Work out the finished part from the listing and answer in its coordinate system (mm). Face numbers are marked on the shaded views. A direction names the side the tool comes from. Coordinates: 2 decimals unless noted, no trailing zeros. Order: outer loops, then holes, each group sorted by start corner. A loop starts at its lowest first (then second) coordinate and runs counter-clockwise, first axis right, second up. Notation, with made-up numbers: M 22.5,-20 L 80.5,-20 A17 cw 80.5,-8 Z; hole C 43,60 d4. An arc over 180 degrees is marked long. Use a Markdown table: item, result.
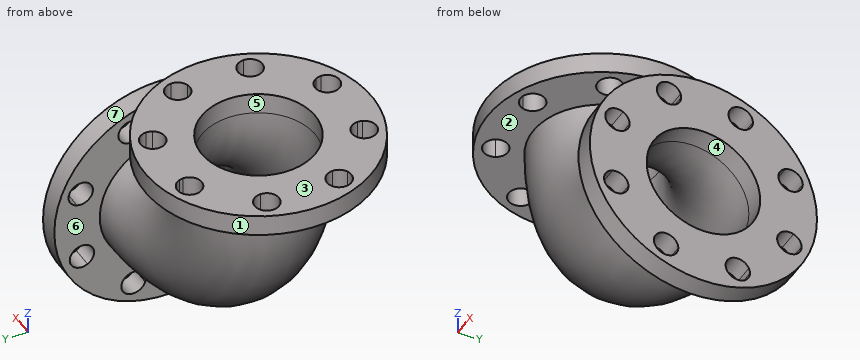
from build123d import *

# Parameters (mm, degrees)
F0_R     = 127
F0_R_2   = 76.2
F0_R_3   = 63.5
F1_DEPTH = 23.8125
F2_ANGLE = 90
F3_R     = 127
F3_R_2   = 76.2
F3_R_3   = 63.5
F4_DEPTH = 23.8125


with BuildPart() as f1:
    # F0 (on Top) → F1 (new body)
    with BuildSketch(Plane.XY):
        Circle(F0_R)
        with BuildLine():
            ThreePointArc((28.8603537964, 100.7217980566), (44.0561876825, 109.567966691), (55.3745369645, 96.1120001135))
            ThreePointArc((55.3745369645, 96.1120001135), (54.9915876268, 92.9004802457), (53.8642145113, 89.8690548525))
            ThreePointArc((53.8642145113, 89.8690548525), (75.3216864654, 72.8316152026), (91.628418296, 50.8137145422))
            ThreePointArc((91.628418296, 50.8137145422), (104.7703861556, 49.9996906202), (111.1174419453, 38.4632770973))
            ThreePointArc((111.1174419453, 38.4632770973), (108.4950074221, 30.41614465), (101.6347694492, 25.4592667608))
            ThreePointArc((101.6347694492, 25.4592667608), (103.9869789782, 12.8260994842), (104.775, 0))
            ThreePointArc((104.775, 0), (103.756751627, -14.5717918189), (100.7217980566, -28.8603537964))
            ThreePointArc((100.7217980565, -28.8603537964), (107.2810644551, -33.856165902), (109.7698250888, -41.7167119892))
            ThreePointArc((109.7698250888, -41.7167119892), (103.2278672199, -53.3743540483), (89.8690548525, -53.8642145113))
            ThreePointArc((89.8690548525, -53.8642145113), (72.8316152026, -75.3216864654), (50.8137145422, -91.628418296))
            ThreePointArc((50.8137145422, -91.628418296), (51.7902477967, -94.4716352042), (52.1211020726, -97.45961697))
            ThreePointArc((52.1211020726, -97.45961697), (40.5762945965, -110.9529983143), (25.4592667608, -101.6347694492))
            ThreePointArc((25.4592667608, -101.6347694492), (-1.7607462756, -104.7602042646), (-28.8603537964, -100.7217980566))
            ThreePointArc((-28.8603537964, -100.7217980566), (-47.1546461423, -108.6405696728), (-53.8642145113, -89.8690548525))
            ThreePointArc((-53.8642145113, -89.8690548525), (-75.3216864654, -72.8316152026), (-91.628418296, -50.8137145422))
            ThreePointArc((-91.628418296, -50.8137145422), (-110.1638535792, -43.4771134759), (-101.6347694492, -25.4592667608))
            ThreePointArc((-101.6347694492, -25.4592667608), (-104.7602042646, 1.7607462756), (-100.7217980566, 28.8603537964))
            ThreePointArc((-100.7217980565, 28.8603537964), (-108.6405696728, 47.1546461423), (-89.8690548525, 53.8642145113))
            ThreePointArc((-89.8690548525, 53.8642145113), (-72.8316152026, 75.3216864654), (-50.8137145422, 91.628418296))
            ThreePointArc((-50.8137145422, 91.628418296), (-43.4771134759, 110.1638535792), (-25.4592667608, 101.6347694492))
            ThreePointArc((-25.4592667608, 101.6347694492), (1.7607462756, 104.7602042646), (28.8603537964, 100.7217980566))
        make_face(mode=Mode.SUBTRACT)
        with BuildLine():
            ThreePointArc((53.8642145113, 89.8690548525), (36.278777836, 83.5834305542), (28.8603537964, 100.7217980566))
            ThreePointArc((28.8603537964, 100.7217980566), (1.7607462756, 104.7602042646), (-25.4592667608, 101.6347694492))
            ThreePointArc((-25.4592667608, 101.6347694492), (-24.969895753, 99.5726344691), (-24.805452122, 97.45961697))
            ThreePointArc((-24.805452122, 97.45961697), (-35.4752953315, 84.1326462706), (-50.8137145422, 91.628418296))
            ThreePointArc((-50.8137145422, 91.628418296), (-72.8316152026, 75.3216864654), (-89.8690548525, 53.8642145113))
            ThreePointArc((-89.8690548525, 53.8642145113), (-84.4543580543, 48.8325790955), (-82.4541751382, 41.7167119892))
            ThreePointArc((-82.4541751382, 41.7167119892), (-88.2514540263, 30.5476476476), (-100.7217980565, 28.8603537964))
            ThreePointArc((-100.7217980566, 28.8603537964), (-104.7602042646, 1.7607462756), (-101.6347694492, -25.4592667608))
            ThreePointArc((-101.6347694492, -25.4592667608), (-89.4124845227, -27.4278866452), (-83.8017919947, -38.4632770973))
            ThreePointArc((-83.8017919947, -38.4632770973), (-85.9232034471, -45.7740462829), (-91.628418296, -50.8137145422))
            ThreePointArc((-91.628418296, -50.8137145422), (-75.3216864654, -72.8316152026), (-53.8642145113, -89.8690548525))
            ThreePointArc((-53.8642145113, -89.8690548525), (-38.5051921214, -82.8371244758), (-28.0588870139, -96.1120001135))
            ThreePointArc((-28.0588870139, -96.1120001135), (-28.2607454116, -98.4514758068), (-28.8603537964, -100.7217980566))
            ThreePointArc((-28.8603537964, -100.7217980566), (-1.7607462756, -104.7602042646), (25.4592667608, -101.6347694492))
            ThreePointArc((25.4592667608, -101.6347694492), (33.4494407187, -84.7553803607), (50.8137145422, -91.628418296))
            ThreePointArc((50.8137145422, -91.628418296), (72.8316152026, -75.3216864654), (89.8690548525, -53.8642145113))
            ThreePointArc((89.8690548525, -53.8642145113), (83.5834305542, -36.278777836), (100.7217980565, -28.8603537964))
            ThreePointArc((100.7217980566, -28.8603537964), (103.756751627, -14.5717918189), (104.775, 0))
            ThreePointArc((104.775, 0), (103.9869789782, 12.8260994842), (101.6347694492, 25.4592667608))
            ThreePointArc((101.6347694492, 25.4592667608), (84.7553803607, 33.4494407187), (91.628418296, 50.8137145422))
            ThreePointArc((91.628418296, 50.8137145422), (75.3216864654, 72.8316152026), (53.8642145113, 89.8690548525))
        make_face()
        Circle(F0_R_2, mode=Mode.SUBTRACT)
        Circle(F0_R_2)
        Circle(F0_R_3, mode=Mode.SUBTRACT)
    extrude(amount=F1_DEPTH)

    # F0 (on Top) → F2 (revolve)
    with BuildSketch(Plane.XY):
        Circle(F0_R_2)
        Circle(F0_R_3, mode=Mode.SUBTRACT)
    revolve(axis=Axis((190.5, -17.9878585041, 0), (0, -1, 0)), revolution_arc=F2_ANGLE)

    # F3 (on face) → F4 (join)
    with BuildSketch(Plane.YZ.offset(190.5)):
        with Locations((0, -190.5)):
            Circle(F3_R)
        with BuildLine():
            ThreePointArc((28.8603537964, -89.7782019434), (44.0561876825, -80.932033309), (55.3745369645, -94.3879998865))
            ThreePointArc((55.3745369645, -94.3879998865), (54.9915876268, -97.5995197543), (53.8642145113, -100.6309451475))
            ThreePointArc((53.8642145113, -100.6309451475), (75.3216864654, -117.6683847974), (91.628418296, -139.6862854578))
            ThreePointArc((91.628418296, -139.6862854578), (104.7703861556, -140.5003093798), (111.1174419453, -152.0367229027))
            ThreePointArc((111.1174419453, -152.0367229027), (108.4950074221, -160.08385535), (101.6347694492, -165.0407332392))
            ThreePointArc((101.6347694492, -165.0407332392), (103.9869789782, -177.6739005158), (104.775, -190.5))
            ThreePointArc((104.775, -190.5), (103.756751627, -205.0717918189), (100.7217980566, -219.3603537964))
            ThreePointArc((100.7217980565, -219.3603537964), (107.2810644551, -224.356165902), (109.7698250888, -232.2167119892))
            ThreePointArc((109.7698250888, -232.2167119892), (103.2278672199, -243.8743540483), (89.8690548525, -244.3642145113))
            ThreePointArc((89.8690548525, -244.3642145113), (72.8316152026, -265.8216864654), (50.8137145422, -282.128418296))
            ThreePointArc((50.8137145422, -282.128418296), (51.7902477967, -284.9716352042), (52.1211020726, -287.95961697))
            ThreePointArc((52.1211020726, -287.95961697), (40.5762945965, -301.4529983143), (25.4592667608, -292.1347694492))
            ThreePointArc((25.4592667608, -292.1347694492), (-1.7607462756, -295.2602042646), (-28.8603537964, -291.2217980566))
            ThreePointArc((-28.8603537964, -291.2217980566), (-47.1546461423, -299.1405696728), (-53.8642145113, -280.3690548525))
            ThreePointArc((-53.8642145113, -280.3690548525), (-75.3216864654, -263.3316152026), (-91.628418296, -241.3137145422))
            ThreePointArc((-91.628418296, -241.3137145422), (-110.1638535792, -233.9771134759), (-101.6347694492, -215.9592667608))
            ThreePointArc((-101.6347694492, -215.9592667608), (-104.7602042646, -188.7392537244), (-100.7217980566, -161.6396462036))
            ThreePointArc((-100.7217980565, -161.6396462036), (-108.6405696728, -143.3453538577), (-89.8690548525, -136.6357854887))
            ThreePointArc((-89.8690548525, -136.6357854887), (-72.8316152026, -115.1783135346), (-50.8137145422, -98.871581704))
            ThreePointArc((-50.8137145422, -98.871581704), (-43.4771134759, -80.3361464208), (-25.4592667608, -88.8652305508))
            ThreePointArc((-25.4592667608, -88.8652305508), (1.7607462756, -85.7397957354), (28.8603537964, -89.7782019434))
        make_face(mode=Mode.SUBTRACT)
        with BuildLine():
            ThreePointArc((53.8642145113, -100.6309451475), (36.278777836, -106.9165694458), (28.8603537964, -89.7782019434))
            ThreePointArc((28.8603537964, -89.7782019434), (1.7607462756, -85.7397957354), (-25.4592667608, -88.8652305508))
            ThreePointArc((-25.4592667608, -88.8652305508), (-24.969895753, -90.9273655309), (-24.805452122, -93.04038303))
            ThreePointArc((-24.805452122, -93.04038303), (-35.4752953315, -106.3673537294), (-50.8137145422, -98.871581704))
            ThreePointArc((-50.8137145422, -98.871581704), (-72.8316152026, -115.1783135346), (-89.8690548525, -136.6357854887))
            ThreePointArc((-89.8690548525, -136.6357854887), (-84.4543580543, -141.6674209045), (-82.4541751382, -148.7832880108))
            ThreePointArc((-82.4541751382, -148.7832880108), (-88.2514540263, -159.9523523524), (-100.7217980565, -161.6396462036))
            ThreePointArc((-100.7217980566, -161.6396462036), (-104.7602042646, -188.7392537244), (-101.6347694492, -215.9592667608))
            ThreePointArc((-101.6347694492, -215.9592667608), (-89.4124845227, -217.9278866452), (-83.8017919947, -228.9632770973))
            ThreePointArc((-83.8017919947, -228.9632770973), (-85.9232034471, -236.2740462829), (-91.628418296, -241.3137145422))
            ThreePointArc((-91.628418296, -241.3137145422), (-75.3216864654, -263.3316152026), (-53.8642145113, -280.3690548525))
            ThreePointArc((-53.8642145113, -280.3690548525), (-38.5051921214, -273.3371244758), (-28.0588870139, -286.6120001135))
            ThreePointArc((-28.0588870139, -286.6120001135), (-28.2607454116, -288.9514758068), (-28.8603537964, -291.2217980566))
            ThreePointArc((-28.8603537964, -291.2217980566), (-1.7607462756, -295.2602042646), (25.4592667608, -292.1347694492))
            ThreePointArc((25.4592667608, -292.1347694492), (33.4494407187, -275.2553803607), (50.8137145422, -282.128418296))
            ThreePointArc((50.8137145422, -282.128418296), (72.8316152026, -265.8216864654), (89.8690548525, -244.3642145113))
            ThreePointArc((89.8690548525, -244.3642145113), (83.5834305542, -226.778777836), (100.7217980565, -219.3603537964))
            ThreePointArc((100.7217980566, -219.3603537964), (103.756751627, -205.0717918189), (104.775, -190.5))
            ThreePointArc((104.775, -190.5), (103.9869789782, -177.6739005158), (101.6347694492, -165.0407332392))
            ThreePointArc((101.6347694492, -165.0407332392), (84.7553803607, -157.0505592813), (91.628418296, -139.6862854578))
            ThreePointArc((91.628418296, -139.6862854578), (75.3216864654, -117.6683847974), (53.8642145113, -100.6309451475))
        make_face()
        with Locations((0, -190.5)):
            Circle(F3_R_2, mode=Mode.SUBTRACT)
        with Locations((0, -190.5)):
            Circle(F3_R_2)
        with Locations((0, -190.5)):
            Circle(F3_R_3, mode=Mode.SUBTRACT)
    extrude(amount=F4_DEPTH)


solid = f1.part
(1) A cutting plane is placed at A-A (y = 0). Determine the outline of the cut face in (x, z), then the cut area to 3 significant figures.
Conclusion:
| item | result |
|---|---|
| outline | M -127,0 L -76.2,0 A266.7 ccw 190.5,-266.7 L 190.5,-317.5 L 214.31,-317.5 L 214.31,-254 L 190.5,-254 A254 cw -63.5,0 L -63.5,23.81 L -127,23.81 Z; M 63.5,0 A127 ccw 190.5,-127 L 214.31,-127 L 214.31,-63.5 L 190.5,-63.5 L 190.5,-114.3 A114.3 cw 76.2,0 L 127,0 L 127,23.81 L 63.5,23.81 Z |
| area | 13,600 mm2 |
(2) A cutting plane is placed at B-B (x = 119.5). Give the number of separate pieces and of enclosed holes in the cut face, then the cut area to 3 significant figures.
Conclusion:
| item | result |
|---|---|
| separate pieces | 2 |
| enclosed holes | 1 |
| area | 8,210 mm2 |
(3) Given P1, Ø6, axis at x = 2.5, z = -77, coming from the -Y side; P2, Ø6, axis at y = -6.5, z = -97, coming from the -X side; P3, Ø8, axis at y = 45, z = -59.5, coming from the +X side, each flat-ended and moving along its own axis, determine where each tip first touches the part or whether it passes through.
Conclusion:
| item | result |
|---|---|
| P1 | y = -75.59 |
| P2 | x = -58.82 |
| P3 | x = 79.85 |
(4) Straight lines are drawn through the part: L1, parallel to Z at x = 206.5, y = 0; L2, parallel to Y at x = -0.5, z = -30; L3, parallel to Y at x = 0, z = 12. For each, find the intervals that lie inside material, in ascending order.
Conclusion:
| item | result |
|---|---|
| L1 | -317.5 to -254, -127 to -63.5 |
| L2 | -76.15 to -63.44, 63.44 to 76.15 |
| L3 | -127 to -63.5, 63.5 to 127 |
(5) Determine the mould class of the marked faces 5, 6 and 7 for opening direction Y: pulls with the +Y half, pulls with the -Y half, needs draft (parallel to the pull), parting line crosses it, or undercut.
Conclusion:
| item | result |
|---|---|
| face 5 | undercut |
| face 6 | needs draft |
| face 7 | parting line crosses it |
(6) Which of the six approach directions +Z, -Z, +X, -X, +Y, -Y give full straight-line access (tool end or side, diameter ignored) to the marked faces 1, 2, 3 and 4?
Conclusion:
| item | result |
|---|---|
| face 1 | +Z |
| face 2 | none |
| face 3 | +Z, +X, -X, +Y, -Y |
| face 4 | +X |
